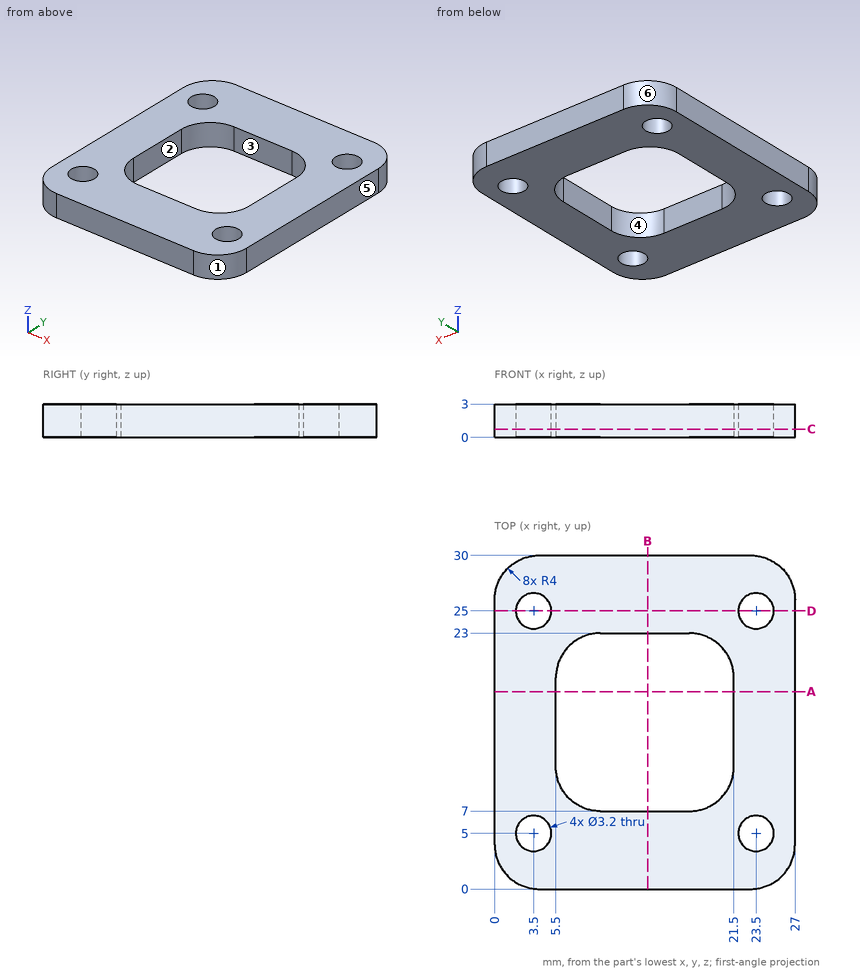
Answer from the drawing. Dimensions are ordinates in mm from the lowest x, y and z of the part. A direction names the side the tool comes from. Give positions to 0.01 mm unless a question says otherwise; leave off trailing zeros. Loops run counter-clockwise (first coordinate to the right, second up) from the corner with the lowest first, then second, coordinate; pieces in that order, holes last.
Item 1: A cutting plane is placed at C-C (z = 0.75). Give the vertices of the cut face in (x, y).
Derived:
outline: (0, 4) arc R4 ccw to (4, 0) - (23, 0) arc R4 ccw to (27, 4) - (27, 26) arc R4 ccw to (23, 30) - (4, 30) arc R4 ccw to (0, 26) - close; hole circle Ø3.2 at (3.5, 5); hole circle Ø3.2 at (3.5, 25); hole (5.5, 11) arc R4 ccw to (9.5, 7) - (17.5, 7) arc R4 ccw to (21.5, 11) - (21.5, 19) arc R4 ccw to (17.5, 23) - (9.5, 23) arc R4 ccw to (5.5, 19) - close; hole circle Ø3.2 at (23.5, 5); hole circle Ø3.2 at (23.5, 25)
Item 2: Each of these flat-tipped pins is pushed along its axis until it touches: pin 1 Ø5 at (x, y) = (23.5, 5) entering from -Z; pin 2 Ø3 at (x, y) = (23.5, 25) entering from -Z; pin 3 Ø1 at (x, z) = (24, 0.5) entering from -Y. Where does it stop, or does it pass through?
Derived:
pin 1: stops at z = 0
pin 2: passes through
pin 3: stops at y = 0.03
Item 3: Determine the mould class of the marked faces 3, 4, 5 and 6 for opening direction Y: +Y half, -Y half, draft (parallel to the pull), parting line (faces both ways), or undercut.
Derived:
face 3: undercut
face 4: undercut
face 5: draft
face 6: +Y half
Item 4: A cutting plane is placed at D-D (y = 25). Give the vertices of the cut face in (x, z).
Derived:
outline: (0, 0) - (1.9, 0) - (1.9, 3) - (0, 3) - close; (5.1, 0) - (21.9, 0) - (21.9, 3) - (5.1, 3) - close; (25.1, 0) - (27, 0) - (27, 3) - (25.1, 3) - close
Item 5: Find the intervals of material crossed by line 1 along Y through (x, z) = (15, 1.5); line 2 along X through (y, z) = (10.75, 1.55); line 3 along Y through (x, z) = (23, 2.55), in increasing order.
Derived:
line 1: y = 0 to 7, 23 to 30
line 2: x = 0 to 5.51, 21.49 to 27
line 3: y = 0 to 3.48, 6.52 to 23.48, 26.52 to 30
Item 6: A cutting plane is placed at B-B (x = 13.75). Give the vertices of the cut face in (y, z).
Derived:
outline: (0, 0) - (7, 0) - (7, 3) - (0, 3) - close; (23, 0) - (30, 0) - (30, 3) - (23, 3) - close
Item 7: A cutting plane is placed at A-A (y = 17.75). Give the vertices of the cut face in (x, z).
Derived:
outline: (0, 0) - (5.5, 0) - (5.5, 3) - (0, 3) - close; (21.5, 0) - (27, 0) - (27, 3) - (21.5, 3) - close
Item 8: A tool of negligible diameter and unlimited length cuts with its end or side. For the marked faces 1 and 2, from which of +Z, -Z, +X, -X, +Y, -Y can it reach the whole face along a straight path? Write none if from no direction.
Derived:
face 1: +Z, -Z, +X, -Y
face 2: +Z, -Z
